Part model, mm, in its own coordinate system. A direction names the side the tool comes from. Give positions to 0.01 mm unless a question says otherwise; leave off trailing zeros. Write each loop counter-clockwise with the first axis right and the second up, starting at its lowest first coordinate (ties: lowest second). Pieces come first, ordered by that corner, then holes. Notation, with made-up numbers: M 89.5,34 L 102.5,34 A20 cw 102.5,47 Z; hole C 63,58 d9. An arc over 180 degrees is marked long. Use a Markdown table: item, result. Add a question column.
from build123d import *

# Parameters (mm, degrees)
SKETCH1_R           = 114.3
SKETCH1_R_2         = 63.5
BOSS_EXTRUDE1_DEPTH = 63.5
SKETCH2_R           = 88.9
SKETCH2_R_2         = 63.5
BOSS_EXTRUDE2_DEPTH = 50.8


with BuildPart() as part:
    # Sketch1 → Boss-Extrude1 (new, symmetric)
    with BuildSketch(Plane(origin=(0, 0, 0), x_dir=(0, 0, -1), z_dir=(1, 0, 0))):
        Circle(SKETCH1_R)
        Circle(SKETCH1_R_2, mode=Mode.SUBTRACT)
    extrude(amount=BOSS_EXTRUDE1_DEPTH, both=True)

    # Sketch2 → Boss-Extrude2 (add)
    with BuildSketch(Plane(origin=(63.5, 0, 0), x_dir=(0, 0, -1), z_dir=(1, 0, 0))):
        Circle(SKETCH2_R)
        Circle(SKETCH2_R_2, mode=Mode.SUBTRACT)
    boss_extrude2 = extrude(amount=BOSS_EXTRUDE2_DEPTH)

    # Mirror1: Boss-Extrude2 across plane
    add(boss_extrude2.mirror(Plane(origin=(0, 0, 0), x_dir=(0, 0, 1), z_dir=(1, 0, 0))))


solid = part.part
1. Mould opens along Y. For faces 4 (the flat face through (114.3, 21, 61)), 5 (the cylindrical face through (1.6, -61.99, 13.77)), 6 (the cylindrical face through (0.89, 5.03, 114.19)) say: released by +Y, released by -Y, zero draft, split by the parting line, or undercut.
2. Flat gauge pins, fed straight in: pin 1 (2 mm diameter, centred on x = 60.5, z = 35, fed in from +Y); pin 2 (8 mm diameter, centred on x = 43.5, z = -47.5, fed in from -Y); pin 3 (2 mm diameter, centred on x = 46.5, y = -82.5, fed in from -Z). Where does each tip first touch, or does it go through?
3. Drill centre lines: probe 1 along Y at (x, z) = (-31, 0); probe 2 along Y at (x, z) = (65, 0); probe 3 along X at (y, z) = (80, -54). Where is each one in solid material? Low to high. Write a range as [from, to].
4. Tool access for faces 1 (the flat face through (-63.5, -67, -59)), 2 (the flat face through (-114.3, 21, 61)), 3 (the cylindrical face through (88.544, 26.703, -84.795)): list every direction of +Z, -Z, +X, -X, +Y, -Y with a clear straight run to the whole face (end or side of a thin tool).
5. Cut at A-A (y = 0). Write the cut outline in (x, z).
6. Cut at D-D (z = 68). Write the cut outline in (x, y).
7. Cut at C-C (x = -90). Write the cut outline in (y, z), then the cut area to 3 significant figures.
A:
| question | item | result |
|---|---|---|
| 1 | face 4 | zero draft |
| 1 | face 5 | undercut |
| 1 | face 6 | split by the parting line |
| 2 | pin 1 | stops at y = 109.13 |
| 2 | pin 2 | stops at y = -105.7 |
| 2 | pin 3 | stops at z = -80.14 |
| 3 | probe 1 | y = [-114.3, -63.5], [63.5, 114.3] |
| 3 | probe 2 | y = [-88.9, -63.5], [63.5, 88.9] |
| 3 | probe 3 | x = [-63.5, 63.5] |
| 4 | face 1 | -X |
| 4 | face 2 | +Z, -Z, -X, +Y, -Y |
| 4 | face 3 | +X |
| 5 | outline | M -114.3,-88.9 L -63.5,-88.9 L -63.5,-114.3 L 63.5,-114.3 L 63.5,-88.9 L 114.3,-88.9 L 114.3,-63.5 L -114.3,-63.5 Z; M -114.3,63.5 L 114.3,63.5 L 114.3,88.9 L 63.5,88.9 L 63.5,114.3 L -63.5,114.3 L -63.5,88.9 L -114.3,88.9 Z |
| 6 | outline | M -114.3,-57.26 L -63.5,-57.26 L -63.5,-91.87 L 63.5,-91.87 L 63.5,-57.26 L 114.3,-57.26 L 114.3,57.26 L 63.5,57.26 L 63.5,91.87 L -63.5,91.87 L -63.5,57.26 L -114.3,57.26 Z |
| 7 | outline | C 0,0 d177.8; hole C 0,0 d127 |
| 7 | area | 12,200 mm² |
